Model file for the job. Use its own axes, mm. Face numbers are marked on the shaded views. A direction names the side the tool comes from. Round coordinates to 2 decimals unless told otherwise and drop trailing zeros. Order: outer loops, then holes, each group sorted by start corner. A loop starts at its lowest first (then second) coordinate and runs counter-clockwise, first axis right, second up. Notation, with made-up numbers: M 42,89 L 97,89 A31 cw 97,128 Z; hole C 23,69.5 d1. An arc over 180 degrees is marked long. Return JSON: item names as keys, results as strings. Group by question number.
Item 1: Slice it at A-A on x = -2. Write the cut outline in (y, z).
Item 2: Pin check, flat tip, straight feed: pin 1 Ø3 at (x, y) = (7.5, -1) entering from +Z. Stop position of the tip, or through.
Item 3: Pull direction Z, two halves, no side cores. Call the marked faces 1, 2 and 3: pulls with the +Z half, pulls with the -Z half, needs draft (parallel to the pull), parting line crosses it, or undercut.
Item 4: Slice it at B-B on x = 7. Write the cut outline in (y, z).
Item 5: Probe line 1 along X through (y, z) = (1.35, 1.8); line 2 along Z through (x, y) = (10.75, 0.4); line 3 along Y through (x, z) = (-1.75, -1). List the from-to ranges inside material, lowest first.
Item 6: Which spindle directions (+Z, -Z, +X, -X, +Y, -Y) get a long thin tool onto all of the face, cutting with end or side? Do the marked faces 4, 5 and 6. Say none if no direction does.
Autodesk Inventor part; units mm, degrees
ref_plane "Work Plane1" through (29, 0, 0) normal (0, -1, 0) x (1, 0, 0)
ref_plane "YZ Plane" through (0, 0, 0) normal (1, 0, 0) x (0, 1, 0)
ref_plane "XZ Plane" through (0, 0, 0) normal (0, 1, 0) x (-1, 0, 0)
sketch "Szkic1" plane through (0, 0, 0) normal (0, 0, 1) x (1, 0, 0)
  line L0 (-0.8667, 0) -> (12, 0)
  line L1 (12, 0) -> (12, 1.5)
  line L2 (12, 1.5) -> (1.25, 1.5)
  line L3 (1.25, 1.5) -> (0.9432, 1.5)
  line L4 (0.9432, 1.5) -> (0, 1.5)
  line L5 (0, 1.5) -> (0, 2.75)
  line L6 (0, 2.75) -> (-3, 2.75)
  line L7 (-3, 2.75) -> (-3, 1.4434)
  line L8 (-3, 1.4434) -> (-1.7, 1.4434)
  line L9 (-1.7, 1.4434) -> (-0.8667, 0)
  line L10 (-6, 0) -> (15, 0)
  line L11 (0, -0.55) -> (0, 3.3)
  line L12 (1.25, 1.5) -> (0, 1.5) construction
  dimension "d1" = 10.75
  dimension "d2" = 0.3068
  dimension "d3" = 3
  dimension "d4" = 1.3
  dimension "d5" = 60
  dimension "d6" = 3
  dimension "d7" = 3
  dimension "d8" = 2.8868
  dimension "d9" = 5.5
  dimension "d26" = 12
revolve "Bryła" add sketch "Szkic1" angle 360 about axis through (-0.8667, 0, 0) along (1, 0, 0)
sketch "Szkic2" plane through (-3, 0, 0) normal (-1, 0, 0) x (0, 0, 1)
  circle A0 centre (0, 0) radius 1.4434
  line L0 (0, -3.85) -> (0, 3.85)
  line L1 (-3.85, 0) -> (3.85, 0)
  line L2 (1.4434, 0) -> (0.7217, -1.25)
  line L3 (0.7217, -1.25) -> (-0.7217, -1.25)
  line L4 (-0.7217, -1.25) -> (-1.4434, 0)
  line L5 (-1.4434, 0) -> (-0.7217, 1.25)
  line L6 (-0.7217, 1.25) -> (0.7217, 1.25)
  line L7 (0.7217, 1.25) -> (1.4434, 0)
  point P0 (0, 0)
extrude "Szczelina" add sketch "Szkic2" against normal up to next contours L7 A0 | A0 L2 | L6 L0 A0 | A0 L0 L3 | L0 L6 A0 | A0 L3 L0 | L4 A0 | A0 L5
fillet "Zaokrąglenie1" radius 0.2 1 edges at (-3, -2.75, 0)
thread "Gwint"
chamfer "Faza1" distance 0.3067 distance2 0.3067 1 edges at (12, -1.5, 0) measured on face at (12, -0.6587, -0.1791)
ref_plane "Work Plane1" through (29, 0, 0) normal (0, -1, 0) x (1, 0, 0)
fillet "Fillet2" radius 0.1 1 edges at (0, -1.5, 0)
equation "\"d1\" = GEL"
equation "\"d3\" = KOH"
equation "\"d4\" = INTI"
equation "\"d6\" = GD"
equation "\"d7\" = BDM"
equation "\"d8\" = 1.1547 * SW"
equation "\"d9\" = KOD"
equation "\"d26\" = NLG"
equation "\"d30\" = R"
equation "\"d17\" = RR"
equation "\"d13\" = GEL"
equation "\"d15\" = -0.5 * SPD + 0.5 * GD"
equation "\"d16\" = GUL"
equation "\"GD\" = NND"
equation "\"NLG\" = 12"
equation "\"GEL\" = 10.75"
equation "\"KOD\" = 5.5"
equation "\"KOH\" = NND"
equation "\"INTI\" = 1.3"
equation "\"GAL\" = 0.61345 * PTC"
equation "\"GUL\" = 0.61345 * PTC"
equation "\"BDM\" = NND"
equation "\"SW\" = 2.5"
equation "\"RR\" = 0.2"
equation "\"SPD\" = NND - 1.2269 * PTC"
equation "\"R\" = 0.1"
equation "\"TOA\" = 30deg"
equation "\"GD1\" = THREADDIA - 1.2269 * PTC"
equation "\"THREADDIA\" = 3"
equation "\"FAWI\" = 45deg"
equation "\"PTC\" = 0.5"
equation "\"NND\" = 3"
equation "\"E0\" = 1.155 * SW"
properties part number "CNS 3932 - M 3 x 12" material "Stal, miękka"
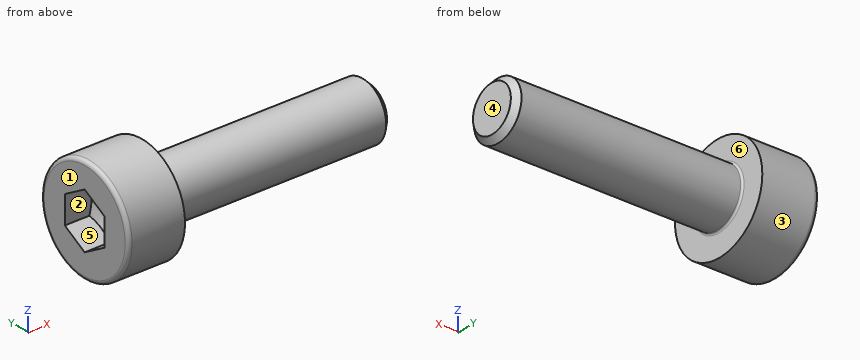
Output values:
{
 "1": {"outline": "C 0,0 d5.5; hole M -1.25,-0.72 L 0,-1.44 L 1.25,-0.72 L 1.25,0.72 L 0,1.44 L -1.25,0.72 Z"},
 "2": {"pin 1": "z = 1.5"},
 "3": {"face 1": "needs draft", "face 2": "undercut", "face 3": "parting line crosses it"},
 "4": {"outline": "C 0,0 d3"},
 "5": {"line 1": "-3 to 0", "line 2": "-1.45 to 1.45", "line 3": "-2.56 to -0.77, 0.77 to 2.56"},
 "6": {"face 4": "+Z, -Z, +X, +Y, -Y", "face 5": "-X", "face 6": "+X"}
}
